Geometry check sheet. Reference: the model listing, model coordinates, mm. A direction names the side the tool comes from. Give positions to 0.01 mm unless a question says otherwise; leave off trailing zeros. Loops run counter-clockwise (first coordinate to the right, second up) from the corner with the lowest first, then second, coordinate; pieces in that order, holes last. Notation, with made-up numbers: (61.25, -5) -> (69.25, -5) arc R21 cw to (69.25, 18) -> close; hole circle Ø3 at (-0.5, 70.5). An arc over 180 degrees is marked (long way). Write item = value, one per line. Start each with the question number.
```python
from build123d import *

# Parameters (mm, degrees)
SHELL1_T                 = -1
BOSS_EXTRUDE2_REACH      = 69.317
BOSS_EXTRUDE2_END_RADIUS = 5.7
BOSS_EXTRUDE2_START      = 5
SKETCH4_W                = 1.5
SKETCH4_H                = 10
CUT_EXTRUDE1_DEPTH       = 1.5
CIRPATTERN1_COUNT        = 4
FILLET1_R                = 0.5


with BuildPart() as part:
    # Sketch2 → Revolve1 (revolve)
    with BuildSketch(Plane.XY, mode=Mode.PRIVATE) as revolve1_sk:
        with BuildLine():
            Line((0, 46.676434016), (-2.777255225, 58.676434016))
            ThreePointArc((-2.777255225, 58.676434016), (-3.833091064, 60.348329411), (-5.7, 61))
            Line((-5.7, 61), (-5.7, 58))
            Line((-5.7, 58), (-5.7, 0))
            Line((-5.7, 0), (0, 0))
            Line((0, 0), (0, 46.676434016))
        make_face()
    revolve(revolve1_sk.sketch.rotate(Axis((-5.7, 58, 0), (0, -1, 0)), 90), axis=Axis((-5.7, 58, 0), (0, -1, 0)))

    # Shell1
    shell1_openings = [part.faces().sort_by_distance(p)[0] for p in [
        (-5.7, 0, 0),
    ]]
    offset(amount=SHELL1_T, openings=shell1_openings, kind=Kind.INTERSECTION)

    # Boss-Extrude2: up to this cylinder (the profile starts outside it)
    boss_extrude2_end = Plane(origin=(-5.7, 5, 0), z_dir=(0, 1, 0)) * Cylinder(BOSS_EXTRUDE2_END_RADIUS, 151.034, mode=Mode.PRIVATE)
    # Sketch4 → Boss-Extrude2 (add, up to the surface)
    with BuildSketch(Plane(origin=(0, 0, 0), x_dir=(0, 0, -1), z_dir=(1, 0, 0)).offset(BOSS_EXTRUDE2_START), mode=Mode.PRIVATE) as boss_extrude2_sk1:
        with Locations((0, 5)):
            Rectangle(SKETCH4_W, SKETCH4_H)
    boss_extrude2_tool1 = extrude(boss_extrude2_sk1.sketch, amount=-BOSS_EXTRUDE2_REACH, mode=Mode.PRIVATE) - boss_extrude2_end
    boss_extrude2 = boss_extrude2_tool1.solids().sort_by_distance((5, 5, 0))[0]
    add(boss_extrude2)

    # Sketch5 → Cut-Extrude1 (cut)
    with BuildSketch(Plane.XY.offset(0.75)):
        Polygon((1, 10), (5, 2), (5, 10), align=None)
    cut_extrude1 = extrude(amount=-CUT_EXTRUDE1_DEPTH, mode=Mode.SUBTRACT)

    # CirPattern1: Boss-Extrude2, Cut-Extrude1 ×4 about axis
    cirpattern1_axis = Axis((-5.7, 0, 0), (0, 1, 0))
    add([boss_extrude2.rotate(cirpattern1_axis, i * 360 / CIRPATTERN1_COUNT) for i in range(1, CIRPATTERN1_COUNT)])
    add([cut_extrude1.rotate(cirpattern1_axis, i * 360 / CIRPATTERN1_COUNT) for i in range(1, CIRPATTERN1_COUNT)], mode=Mode.SUBTRACT)

    # Fillet1
    fillet1_edges = [part.edges().sort_by_distance(p)[0] for p in [
        (-0.049557539, 5, -0.75),
        (0.47522123, 10, -0.75),
        (0, 10, 0),
        (0.47522123, 10, 0.75),
        (-0.049557539, 5, 0.75),
        (1, 10, 0),
        (-6.45, 5, -5.650442461),
        (-6.45, 10, -6.17522123),
        (-5.7, 10, -5.7),
        (-4.95, 10, -6.17522123),
        (-4.95, 5, -5.650442461),
        (-11.350442461, 5, 0.75),
        (-11.87522123, 10, 0.75),
        (-11.4, 10, 0),
        (-11.87522123, 10, -0.75),
        (-11.350442461, 5, -0.75),
        (-6.45, 5, 5.650442461),
        (-5.324182242, 10, 5.687597121),
        (-6.45, 10, 6.17522123),
        (-4.95, 5, 5.650442461),
        (-4.95, 10, 6.17522123),
        (-5.7, 10, -6.7),
        (-12.4, 10, 0),
        (-5.7, 10, 6.7),
    ]]
    fillet(fillet1_edges, radius=FILLET1_R)


solid = part.part
```
1) Thickness scan on line 1 (X direction, y = 20, z = 0); line 2 (Y direction, x = -12, z = -0.25); line 3 (X direction, y = 36, z = -2.5). Record the ranges inside material, lowest first.
2) Section check A-A (y = 4). Enter the section's corners in (x, z), plus the area to 3 significant figures.
3) Draft check along X on faces 5 (the flat face through (-6.45, 4, -8)), 6 (the cylindrical face through (-9.66, 23.61, 2.53)), 7 (the flat face through (-4.95, 4, 8)). Enter one of: released by +X, released by -X, zero draft, split by the parting line, or undercut.
4) Tool access check on faces 1 (the flat face through (2, 4, 0.75)), 2 (the flat face through (2, 4, -0.75)), 3 (the flat face through (-6.45, 4, 8)), 4 (the flat face through (-14, 4, -0.75)). Record the directions out of +Z, -Z, +X, -X, +Y, -Y that give a thin tool (end or side, any length) a straight path to the whole face; none if there is none.
5) Depth check by flat-ended pin: pin 1 Ø8 at (y, z) = (23.5, 4.5) entering from -X; pin 2 Ø3.5 at (x, y) = (2, 4) entering from -Z; pin 3 Ø3.5 at (x, y) = (2, 6) entering from +Z; pin 4 Ø1.5 at (y, z) = (46.5, 7) entering from +X. Enter the tip coordinate at first touch or a pass-through.
6) Section check B-B (z = 8). Enter the section's corners in (x, y).
7) Section check C-C (y = 15). Enter the section's corners in (x, z), plus the area to 3 significant figures.
8) Section check D-D (z = -8.25). Enter the section's corners in (x, y).
Check result:
q1.line_1 = -11.4 to -10.4, -1 to 0
q1.line_2 = 0 to 10
q1.line_3 = -10.82 to -9.68, -1.72 to -0.58
q2.outline = (-15.4, -0.75) -> (-11.77, -0.75) arc R0.5 cw to (-11.28, -1.15) arc R5.7 ccw to (-6.85, -5.58) arc R0.5 cw to (-6.45, -6.07) -> (-6.45, -9.7) -> (-4.95, -9.7) -> (-4.95, -6.07) arc R0.5 cw to (-4.55, -5.58) arc R5.7 ccw to (-0.12, -1.15) arc R0.5 cw to (0.37, -0.75) -> (4, -0.75) -> (4, 0.75) -> (0.37, 0.75) arc R0.5 cw to (-0.12, 1.15) arc R5.7 ccw to (-4.55, 5.58) arc R0.5 cw to (-4.95, 6.07) -> (-4.95, 9.7) -> (-6.45, 9.7) -> (-6.45, 6.07) arc R0.5 cw to (-6.85, 5.58) arc R5.7 ccw to (-11.28, 1.15) arc R0.5 cw to (-11.77, 0.75) -> (-15.4, 0.75) -> close; hole circle Ø9.4 at (-5.7, 0)
q2.area = 57.0 mm2
q3.face_5 = released by -X
q3.face_6 = undercut
q3.face_7 = released by +X
q4.face_1 = +Z, +X, +Y, -Y
q4.face_2 = -Z, +X, +Y, -Y
q4.face_3 = +Z, -X, +Y, -Y
q4.face_4 = -Z, -X, +Y, -Y
q5.pin_1 = -11.38
q5.pin_2 = -0.77
q5.pin_3 = 0.77
q5.pin_4 = through
q6.outline = (-6.45, 0) -> (-4.95, 0) -> (-4.95, 7.4) -> (-6.45, 7.4) -> close
q7.outline = circle Ø11.4 at (-5.7, 0); hole circle Ø9.4 at (-5.7, 0)
q7.area = 32.7 mm2
q8.outline = (-6.45, 0) -> (-4.95, 0) -> (-4.95, 6.9) -> (-6.45, 6.9) -> close
